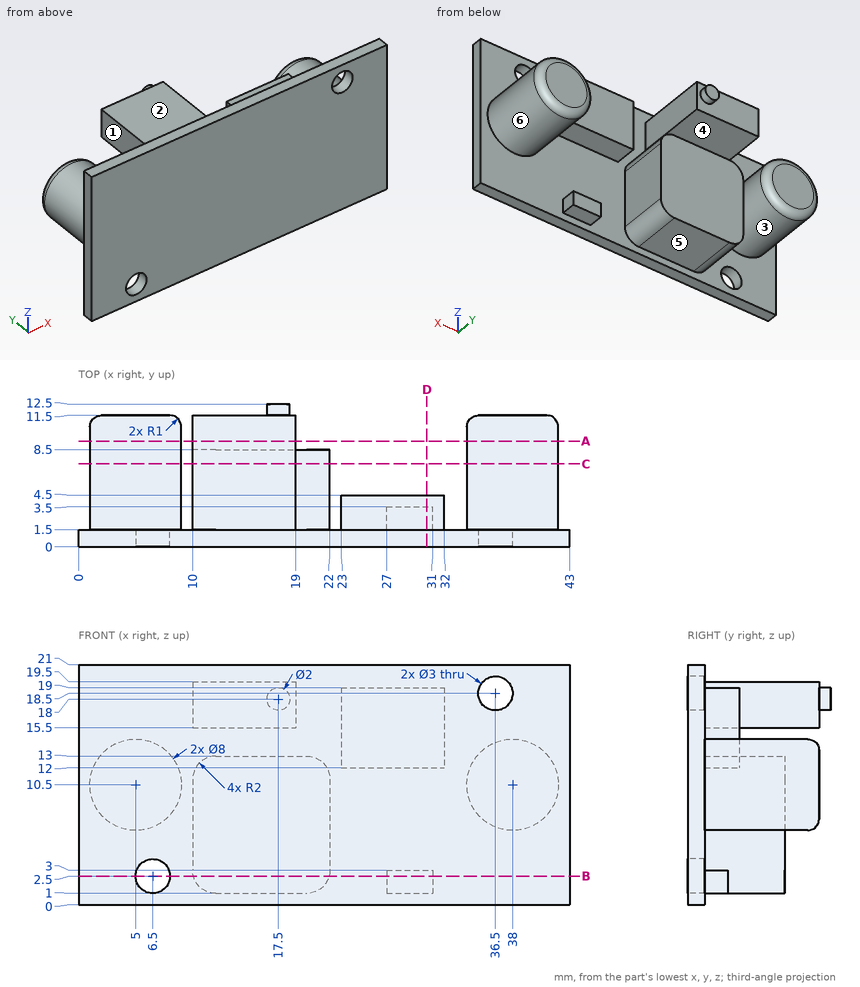
The drawing under review shows one solid part. Ordinate dimensions are in mm from its lowest x, y, z. A direction names the side the tool comes from. Coordinates: 2 decimals unless noted, no trailing zeros. Order: outer loops, then holes, each group sorted by start corner. A loop starts at its lowest first (then second) coordinate and runs counter-clockwise, first axis right, second up. Notation, with made-up numbers: (52, 74.5) -> (83, 74.5) arc R13 ccw to (83, 96.5) -> close; hole circle Ø4 at (5, 35). An arc over 180 degrees is marked (long way). Answer in a Markdown table with one row per item.
(1) Wall thickness on line 1 along Z through (x, y) = (6.5, 0.95); line 2 along X through (y, z) = (0.55, 18.5); line 3 along Z through (x, y) = (16.5, 3): over which ranges is each line inside the solid? List them lowest first.
Answers:
| item | result |
|---|---|
| line 1 | 0 to 1, 4 to 21 |
| line 2 | 0 to 35, 38 to 43 |
| line 3 | 1 to 13, 15.5 to 19.5 |
(2) Consider section C-C (y = 7.25). Write out the cut boundary in (x, z), plus the area to 3 significant figures.
Answers:
| item | result |
|---|---|
| outline | circle Ø8 at (5, 10.5); (10, 3) arc R2 ccw to (12, 1) -> (20, 1) arc R2 ccw to (22, 3) -> (22, 11) arc R2 ccw to (20, 13) -> (12, 13) arc R2 ccw to (10, 11) -> close; (10, 15.5) -> (19, 15.5) -> (19, 19.5) -> (10, 19.5) -> close; circle Ø8 at (38, 10.5) |
| area | 277 mm² |
(3) The part is to be moulded in two halves that separate along X. For the marked faces 1, 2 and 3, say which applies: +X half, -X half, draft (parallel to the pull), parting line (faces both ways), or undercut.
Answers:
| item | result |
|---|---|
| face 1 | -X half |
| face 2 | draft |
| face 3 | undercut |
(4) Consider section D-D (x = 30.5). Write out the cut boundary in (y, z).
Answers:
| item | result |
|---|---|
| outline | (0, 0) -> (1.5, 0) -> (1.5, 1) -> (3.5, 1) -> (3.5, 3) -> (1.5, 3) -> (1.5, 12) -> (4.5, 12) -> (4.5, 19) -> (1.5, 19) -> (1.5, 21) -> (0, 21) -> close |
(5) Insertion check: pin 1 (5 mm diameter, centred on x = 36.5, z = 18.5, fed in from +Y); pin 2 (1.2 mm diameter, centred on y = 7.5, z = 17.5, fed in from -X); pin 3 (2 mm diameter, centred on x = 15.5, y = 6.5, fed in from +Z). Each pin has a flat end and moves straight along its axis. Give the tip position at first contact, or say it passes through.
Answers:
| item | result |
|---|---|
| pin 1 | y = 1.5 |
| pin 2 | x = 10 |
| pin 3 | z = 19.5 |
(6) Consider section A-A (y = 9.25). Write out the cut boundary in (x, z).
Answers:
| item | result |
|---|---|
| outline | circle Ø8 at (5, 10.5); (10, 15.5) -> (19, 15.5) -> (19, 19.5) -> (10, 19.5) -> close; circle Ø8 at (38, 10.5) |
(7) Machinability: for the marked faces 4, 5 and 6, which of the approach directions +Z, -Z, +X, -X, +Y, -Y give a long, thin tool a straight path to every point of the face, cutting with its end or side? Answer none if there is none.
Answers:
| item | result |
|---|---|
| face 4 | -X, +Y |
| face 5 | -Z, +X, -X, +Y |
| face 6 | +Y |
(8) Consider section B-B (z = 2.5). Write out the cut boundary in (x, y).
Answers:
| item | result |
|---|---|
| outline | (0, 0) -> (5, 0) -> (5, 1.5) -> (0, 1.5) -> close; (8, 0) -> (43, 0) -> (43, 1.5) -> (31, 1.5) -> (31, 3.5) -> (27, 3.5) -> (27, 1.5) -> (21.94, 1.5) -> (21.94, 8.5) -> (10.06, 8.5) -> (10.06, 1.5) -> (8, 1.5) -> close |
